Geometry check sheet. Reference: drawing and pictorial views, mm from the part's lowest x, y, z. A direction names the side the tool comes from. Coordinates: 2 decimals unless noted, no trailing zeros. Loops run counter-clockwise (first coordinate to the right, second up) from the corner with the lowest first, then second, coordinate; pieces in that order, holes last. Notation, with made-up numbers: M 34,62.5 L 79,62.5 A31 cw 79,86.5 Z; hole C -33.75,27 d9. An arc over 180 degrees is marked long. Write item = value, one per line. Start each with the question number.
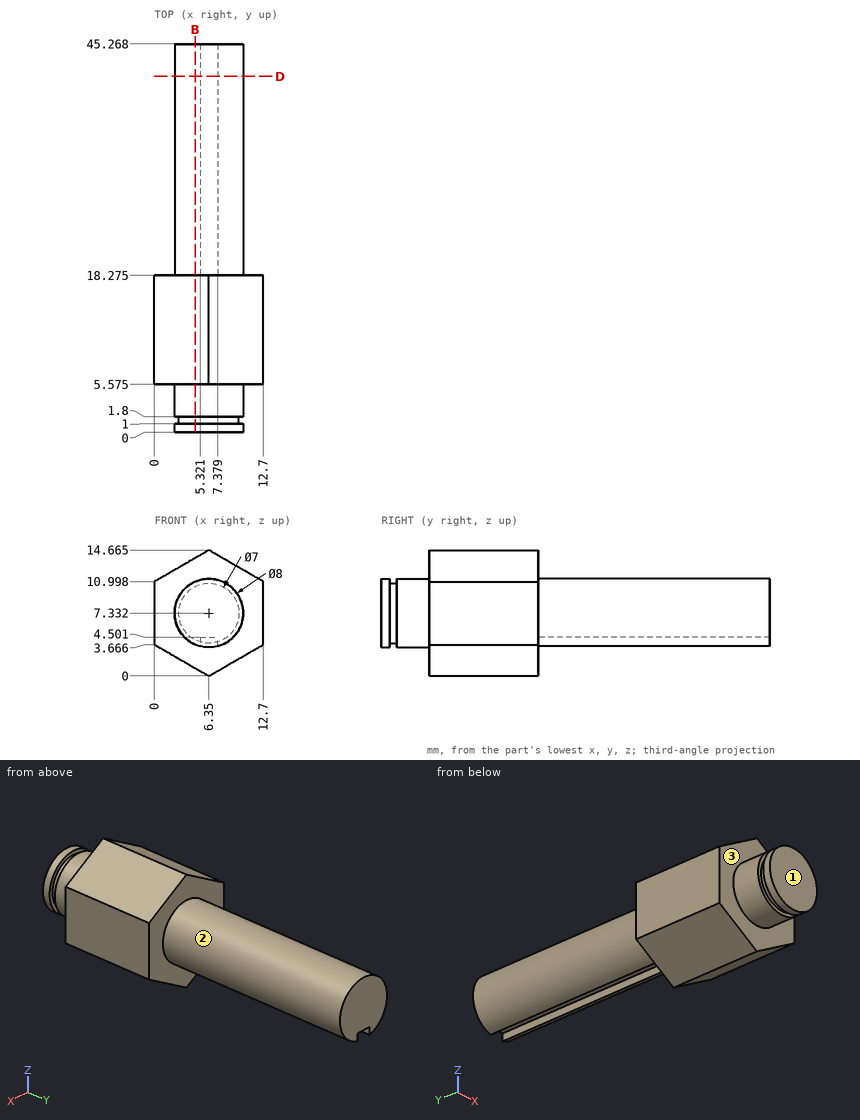
Q1. Sectioned sample at D-D on y = 41.5. Record the cut outline in (x, z).
Q2. Gauge pin test, flat ends, axial feed: pin 1 (4 mm diameter, centred on x = 5.5, z = 6, fed in from -Y); pin 2 (2 mm diameter, centred on x = 4.5, y = 32, fed in from +Z); pin 3 (1.1 mm diameter, centred on y = 37, z = 4, fed in from -X) (1 decimal); pin 4 (1.1 mm diameter, centred on y = 34.5, z = 4, fed in from +X) (1 decimal). Record the tip position at first contact, or that the pin passes through.
Q3. Scan lines: L1, parallel to Y at x = 8.75, z = 10; L2, parallel to Y at x = 2.25, z = 4 (1 decimal); L3, parallel to X at y = 32, z = 4 (1 decimal). Record each from-to range of solid material in increasing order. Write a range as [from, to].
Q4. Sectioned sample at B-B on x = 4.75. Record the cut outline in (y, z) (1 decimal).
Q5. Set-up check for the marked faces 1, 2 and 3: record each of +Z, -Z, +X, -X, +Y, -Y from which the full face is reachable in a straight line by a thin tool's end or side.
Solutions:
q1.outline = M 5.32,3.47 L 5.32,4.5 L 7.38,4.5 L 7.38,3.47 A4 ccw long Z
q2.pin_1 = 0
q2.pin_2 = 11.24
q2.pin_3 = 3.5
q2.pin_4 = 9.2
q3.L1 = [0, 1], [1.8, 45.27]
q3.L2 = [5.6, 18.3]
q3.L3 = [4.1, 5.3], [7.4, 8.6]
q4.outline = M 0,3.7 L 1,3.7 L 1,4.2 L 1.8,4.2 L 1.8,3.7 L 5.6,3.7 L 5.6,0.9 L 18.3,0.9 L 18.3,3.7 L 45.3,3.7 L 45.3,11 L 18.3,11 L 18.3,13.7 L 5.6,13.7 L 5.6,11 L 1.8,11 L 1.8,10.4 L 1,10.4 L 1,11 L 0,11 Z
q5.face_1 = +Z, -Z, +X, -X, -Y
q5.face_2 = +Y
q5.face_3 = -Y
